```python
from build123d import *

# Parameters (mm, degrees)
SKETCH1_R                = 60.325
SKETCH1_R_2              = 4.064
BOSS_EXTRUDE1_DEPTH      = 5.08
BOSS_EXTRUDE2_DEPTH      = 6.35
BOSS_EXTRUDE2_DEPTH_BACK = 247.65
SKETCH2_R                = 9.525
SKETCH4_W                = 4.318
SKETCH4_H                = 2.15
CUT_EXTRUDE1_DEPTH       = 228.6


with BuildPart() as part:
    # Sketch1 → Boss-Extrude1 (new body)
    with BuildSketch(Plane(origin=(0, 0, 0), x_dir=(0, 0, -1), z_dir=(1, 0, 0))):
        Circle(SKETCH1_R)
        with Locations((0, -50.292)):
            Circle(SKETCH1_R_2, mode=Mode.SUBTRACT)
        with Locations((-47.830534318, -15.541082681)):
            Circle(SKETCH1_R_2, mode=Mode.SUBTRACT)
        with Locations((-29.560895908, 40.687082681)):
            Circle(SKETCH1_R_2, mode=Mode.SUBTRACT)
        with Locations((29.560895908, 40.687082681)):
            Circle(SKETCH1_R_2, mode=Mode.SUBTRACT)
        with Locations((47.830534318, -15.541082681)):
            Circle(SKETCH1_R_2, mode=Mode.SUBTRACT)
    extrude(amount=BOSS_EXTRUDE1_DEPTH)

    # Sketch2 → Boss-Extrude2 (add, two sides: drawn at the far end of the back side and taken through both)
    with BuildSketch(Plane(origin=(5.08, 0, 0), x_dir=(0, 0, -1), z_dir=(1, 0, 0)).offset(-BOSS_EXTRUDE2_DEPTH_BACK)):
        Circle(SKETCH2_R)
    extrude(amount=BOSS_EXTRUDE2_DEPTH + BOSS_EXTRUDE2_DEPTH_BACK)

    # Sketch4 → Cut-Extrude1 (cut)
    with BuildSketch(Plane.ZY.offset(242.57)):
        with Locations((0, 8.45)):
            Rectangle(SKETCH4_W, SKETCH4_H)
    extrude(amount=-CUT_EXTRUDE1_DEPTH, mode=Mode.SUBTRACT)


solid = part.part
```
The listing builds one solid part. Answer for the finished solid, in the listing's coordinates (mm). A direction names the side the tool comes from. Give positions to 0.01 mm unless a question says otherwise; leave off trailing zeros. Loops run counter-clockwise (first coordinate to the right, second up) from the corner with the lowest first, then second, coordinate; pieces in that order, holes last. Notation, with made-up numbers: M 78.5,69.25 L 96.5,69.25 A20 ccw 96.5,100.25 Z; hole C -15,-32 d1. An arc over 180 degrees is marked long. One line per item, written item: value.
Q1. A cutting plane is placed at A-A on y = 0. Determine the outline of the cut face in (x, z) (3 decimals).
Working result:
outline: M -242.57,-9.525 L 0,-9.525 L 0,-60.325 L 5.08,-60.325 L 5.08,-9.525 L 11.43,-9.525 L 11.43,9.525 L 5.08,9.525 L 5.08,60.325 L 0,60.325 L 0,9.525 L -242.57,9.525 Z
Q2. A cutting plane is placed at C-C on z = -17.5. Determine the outline of the cut face in (x, y), then the cut area to 3 significant figures.
Working result:
outline: M 0,-57.73 L 5.08,-57.73 L 5.08,57.73 L 0,57.73 Z
area: 587 mm^2
Q3. For faces 1 (the face through (-122.98, -9.3, 2.06)), 2 (the face through (8.211, -5.796, 7.559)), 3 (the face through (2.5, 36.72, -28.68)), determine the directions among +Z, -Z, +X, -X, +Y, -Y from which every point of the face is accessible in a straight line to the end or side of a thin tool.
Working result:
face 1: -X
face 2: +X
face 3: +X, -X
Q4. Flat-ended cylindrical pins translate along their axes: P1, Ø1.1, axis at y = 9, z = 0, coming from the -X side; P2, Ø10.5, axis at y = -50.292, z = 0, coming from the -X side; P3, Ø4.5, axis at x = -125.5, z = 0, coming from the +Y side. Find the tip coordinate at first contact, or state that the pin passes through.
Working result:
P1: stops at x = -13.97
P2: stops at x = 0
P3: stops at y = 9.28
Q5. A cutting plane is placed at B-B on x = -221. Determine the outline of the cut face in (y, z) (3 decimals), then the cut area to 3 significant figures.
Working result:
outline: M 7.375,-2.159 L 7.375,2.159 L 9.277,2.159 A9.525 ccw long 9.277,-2.159 Z
area: 276 mm^2
Q6. Determine the mould class of faces 4 (the face through (2.504, 2.652, 60.267)), 5 (the face through (2.5, -15.36, 51.89)), 6 (the face through (11.43, 0, 0)) for opening direction Y: +Y half, -Y half, draft (parallel to the pull), parting line (faces both ways), or undercut.
Working result:
face 4: parting line
face 5: undercut
face 6: draft
Q7. Find the intervals of material crossed by line 1 (Y direction, x = 2.15, z = 0) (3 decimals); line 2 (X direction, y = -11, z = -21); line 3 (Z direction, x = -44, y = 0.5), in increasing order. Write a range as from..to.
Working result:
line 1: y = -60.325..-54.356, -46.228..60.325
line 2: x = 0..5.08
line 3: z = -9.51..9.51
